```python
from build123d import *

# Parameters (mm, degrees)
BOSS_EXTRUDE1_DEPTH = 50.8
SKETCH4_W           = 2
SKETCH4_H           = 28.319341289
BOSS_EXTRUDE2_DEPTH = 10
SKETCH5_W           = 5
SKETCH5_H           = 28.319341289
CUT_EXTRUDE2_DEPTH  = 1
SKETCH8_R           = 14
CUT_EXTRUDE3_DEPTH  = 70.841706276


with BuildPart() as part:
    # Sketch1 → Boss-Extrude1 (new body)
    with BuildSketch(Plane(origin=(0, 0, 0), x_dir=(1, 0, 0), z_dir=(0, 1, 0))):
        with BuildLine():
            Line((-46.87455531, -10.750952702), (46.87455531, -10.750952702))
            ThreePointArc((46.87455531, -10.750952702), (43.857336275, -8.175639398), (40, -7.250001141))
            Line((40, -7.250001141), (-40, -7.250001141))
            ThreePointArc((-40, -7.250001141), (-43.857336275, -8.175639398), (-46.87455531, -10.750952702))
        make_face()
    extrude(amount=BOSS_EXTRUDE1_DEPTH)

    # Sketch4 → Boss-Extrude2 (add)
    with BuildSketch(Plane.XY.offset(10.750952702)):
        with Locations((41.6, 24.891155304)):
            Rectangle(SKETCH4_W, SKETCH4_H)
    boss_extrude2 = extrude(amount=BOSS_EXTRUDE2_DEPTH)

    # Sketch5 → Cut-Extrude2 (cut)
    with BuildSketch(Plane(origin=(42.6, 0, 0), x_dir=(0, 0, -1), z_dir=(1, 0, 0))):
        with Locations((-13.250952702, 24.891155304)):
            Rectangle(SKETCH5_W, SKETCH5_H)
    cut_extrude2 = extrude(amount=-CUT_EXTRUDE2_DEPTH, mode=Mode.SUBTRACT)

    # Mirror1: Boss-Extrude2, Cut-Extrude2 across plane
    add(boss_extrude2.mirror(Plane(origin=(0, 0, 0), x_dir=(0, 0, 1), z_dir=(1, 0, 0))))
    add(cut_extrude2.mirror(Plane(origin=(0, 0, 0), x_dir=(0, 0, 1), z_dir=(1, 0, 0))), mode=Mode.SUBTRACT)

    # Sketch8 → Cut-Extrude3 (cut, through all)
    with BuildSketch(Plane.XY.offset(10.750952702)):
        with Locations((0, 25.5)):
            Circle(SKETCH8_R)
    extrude(amount=-CUT_EXTRUDE3_DEPTH, mode=Mode.SUBTRACT)


solid = part.part
```
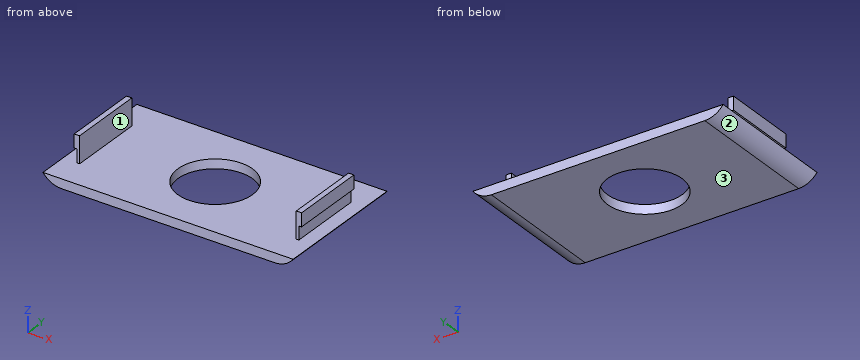
Geometry: final body of the model. Coordinates: model frame, mm. Face numbers are marked on the shaded views. Round coordinates to 2 decimals unless told otherwise and drop trailing zeros. Loops run counter-clockwise (first coordinate to the right, second up) from the corner with the lowest first, then second, coordinate; pieces in that order, holes last. Notation, with made-up numbers: (84, -20) -> (132, -20) arc R21 ccw to (132, 7) -> close; hole circle Ø8 at (16.5, 4). An arc over 180 degrees is marked (long way). Use one line per item in the form item = value. Start each with the question number.
1) Section D-D on y = 32. Output: boundary loops of the cut face in (x, z).
2) Section A-A on z = 13. Output: boundary loops of the cut face in (x, y).
3) First-contact query: P1, Ø2, axis at x = -42, z = 16, coming from the +Y side; P2, Ø3, axis at y = 16, z = 17.5, coming from the -X side; P3, Ø2, axis at x = 2, y = 45.5, coming from the +Z side; P4, Ø22.5, axis at x = 0, y = 25.5, coming from the -Z side. Flat tips, straight axial feed; report the tip coordinate or a pass-through.
4) Line query: L1, parallel to Y at x = 0, z = 9.3; L2, parallel to X at y = 26, z = 17.75; L3, parallel to Z at x = 0, y = 10.5. Output: solid intervals per line, ascending.
5) Draft query along X for the marked faces 1, 2 and 3. Return one class per face: released by +X, released by -X, zero draft, split by the parting line, or undercut.
6) Section C-C on x = 0. Output: boundary loops of the cut face in (y, z).
7) Section B-B on y = 26.5. Output: boundary loops of the cut face in (x, z).
Response:
q1.outline = (-46.87, 10.75) arc R8.5 ccw to (-40, 7.25) -> (-12.4, 7.25) -> (-12.4, 10.75) -> (-40.6, 10.75) -> (-40.6, 20.75) -> (-42.6, 20.75) -> (-42.6, 15.75) -> (-41.6, 15.75) -> (-41.6, 10.75) -> close; (12.4, 7.25) -> (40, 7.25) arc R8.5 ccw to (46.87, 10.75) -> (41.6, 10.75) -> (41.6, 15.75) -> (42.6, 15.75) -> (42.6, 20.75) -> (40.6, 20.75) -> (40.6, 10.75) -> (12.4, 10.75) -> close
q2.outline = (-41.6, 10.73) -> (-40.6, 10.73) -> (-40.6, 39.05) -> (-41.6, 39.05) -> close; (40.6, 10.73) -> (41.6, 10.73) -> (41.6, 39.05) -> (40.6, 39.05) -> close
q3.P1 = 39.05
q3.P2 = -42.6
q3.P3 = 10.75
q3.P4 = through
q4.L1 = 0 to 11.5, 39.5 to 50.8
q4.L2 = -42.6 to -40.6, 40.6 to 42.6
q4.L3 = 7.25 to 10.75
q5.face_1 = undercut
q5.face_2 = released by -X
q5.face_3 = zero draft
q6.outline = (0, 7.25) -> (11.5, 7.25) -> (11.5, 10.75) -> (0, 10.75) -> close; (39.5, 7.25) -> (50.8, 7.25) -> (50.8, 10.75) -> (39.5, 10.75) -> close
q7.outline = (-46.87, 10.75) arc R8.5 ccw to (-40, 7.25) -> (-13.96, 7.25) -> (-13.96, 10.75) -> (-40.6, 10.75) -> (-40.6, 20.75) -> (-42.6, 20.75) -> (-42.6, 15.75) -> (-41.6, 15.75) -> (-41.6, 10.75) -> close; (13.96, 7.25) -> (40, 7.25) arc R8.5 ccw to (46.87, 10.75) -> (41.6, 10.75) -> (41.6, 15.75) -> (42.6, 15.75) -> (42.6, 20.75) -> (40.6, 20.75) -> (40.6, 10.75) -> (13.96, 10.75) -> close
